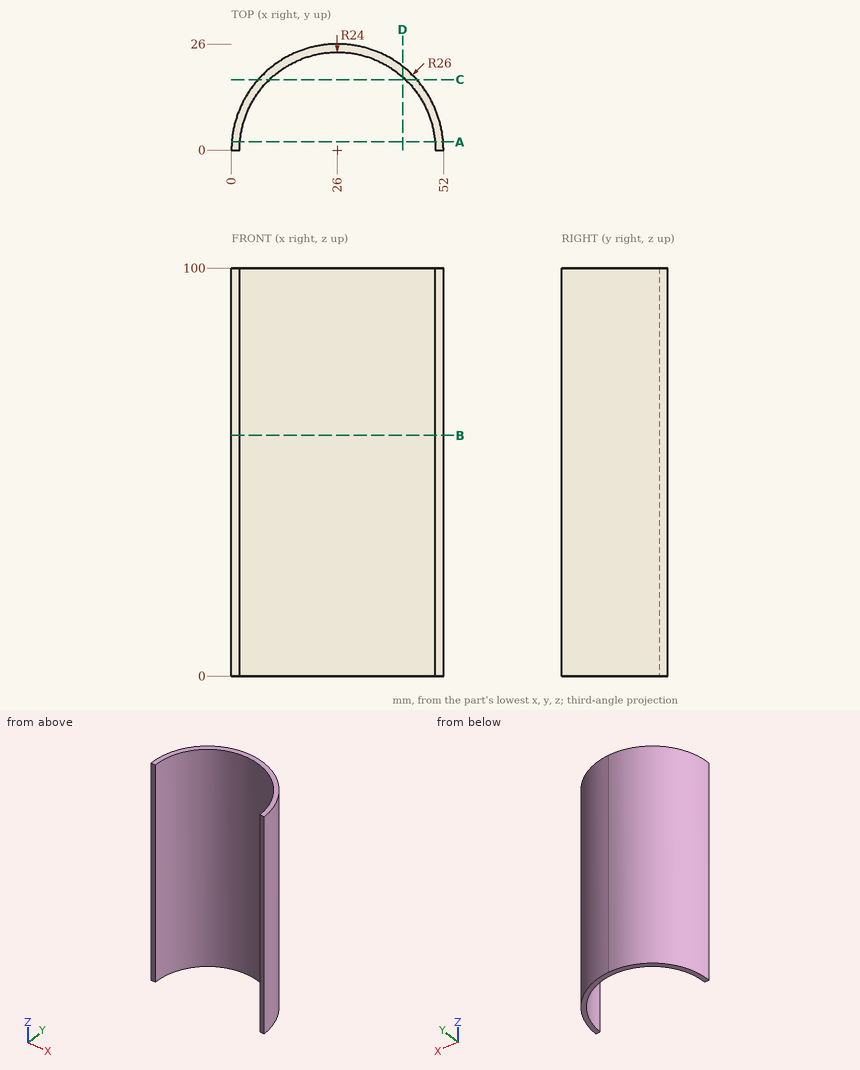
The drawing under review shows one solid part. Ordinate dimensions are in mm from its lowest x, y, z. Coordinates: 2 decimals unless noted, no trailing zeros. Write each loop counter-clockwise with the first axis right and the second up, starting at its lowest first coordinate (ties: lowest second). Pieces come first, ordered by that corner, then holes. Notation, with made-up numbers: (21.25, 54.25) -> (65.25, 54.25) arc R34 ccw to (65.25, 88.25) -> close; hole circle Ø1 at (-33, 62.5). An arc over 180 degrees is marked (long way). Write each question's results on one line, items separated by ' | '. Start each with the question number.
1) Insertion check: pin 1 (8 mm diameter, centred on x = 15, z = 70, fed in from +Y); pin 2 (2 mm diameter, centred on y = 9.5, z = 68, fed in from +X); pin 3 (1 mm diameter, centred on y = 8.5, z = 36, fed in from +X); pin 4 (10 mm diameter, centred on x = 20, y = 20.5, fed in from -Z). Each pin has a flat end and moves straight along its axis. Give the tip position at first contact, or say it passes through.
2) Wall thickness on L1, parallel to X at y = 15, z = 46 (3 decimals); L2, parallel to Y at x = 25.5, z = 75.5; L3, parallel to X at y = 13, z = 57.5: over which ranges is each line inside the solid? List them lowest first. Write a range as [from, to].
3) Consider section B-B (z = 59). Write out the cut boundary in (x, y), plus the area to 3 significant figures.
4) Consider section C-C (y = 17.25). Write out the cut boundary in (x, z).
5) Consider section D-D (x = 42). Write out the cut boundary in (y, z), plus the area to 3 significant figures.
6) Consider section A-A (y = 2). Write out the cut boundary in (x, z), plus the area to 3 significant figures.
Geometry says:
1) pin 1: y = 25.04 | pin 2: x = 50.57 | pin 3: x = 50.74 | pin 4: z = 0
2) L1: [4.763, 7.265], [44.735, 47.237] | L2: [23.99, 26] | L3: [3.48, 5.83], [46.17, 48.52]
3) outline: (0, 0) -> (2, 0) arc R24 cw to (50, 0) -> (52, 0) arc R26 ccw to start | area: 157 mm^2
4) outline: (6.55, 0) -> (9.31, 0) -> (9.31, 100) -> (6.55, 100) -> close; (42.69, 0) -> (45.45, 0) -> (45.45, 100) -> (42.69, 100) -> close
5) outline: (17.89, 0) -> (20.49, 0) -> (20.49, 100) -> (17.89, 100) -> close | area: 261 mm^2
6) outline: (0.08, 0) -> (2.08, 0) -> (2.08, 100) -> (0.08, 100) -> close; (49.92, 0) -> (51.92, 0) -> (51.92, 100) -> (49.92, 100) -> close | area: 401 mm^2
